For this review, use the dimensioned drawing (mm, ordinates from the lowest corner) and the shaded views. Give positions to 0.01 mm unless a question says otherwise; leave off trailing zeros. Write each loop counter-clockwise with the first axis right and the second up, starting at its lowest first coordinate (ties: lowest second). Pieces come first, ordered by that corner, then holes. Notation, with made-up numbers: M 16,14 L 24,14 A26 cw 24,43 Z; hole C 87.25,13 d9. An arc over 180 degrees is marked long. Use a Markdown table: item, result. Add a question column.
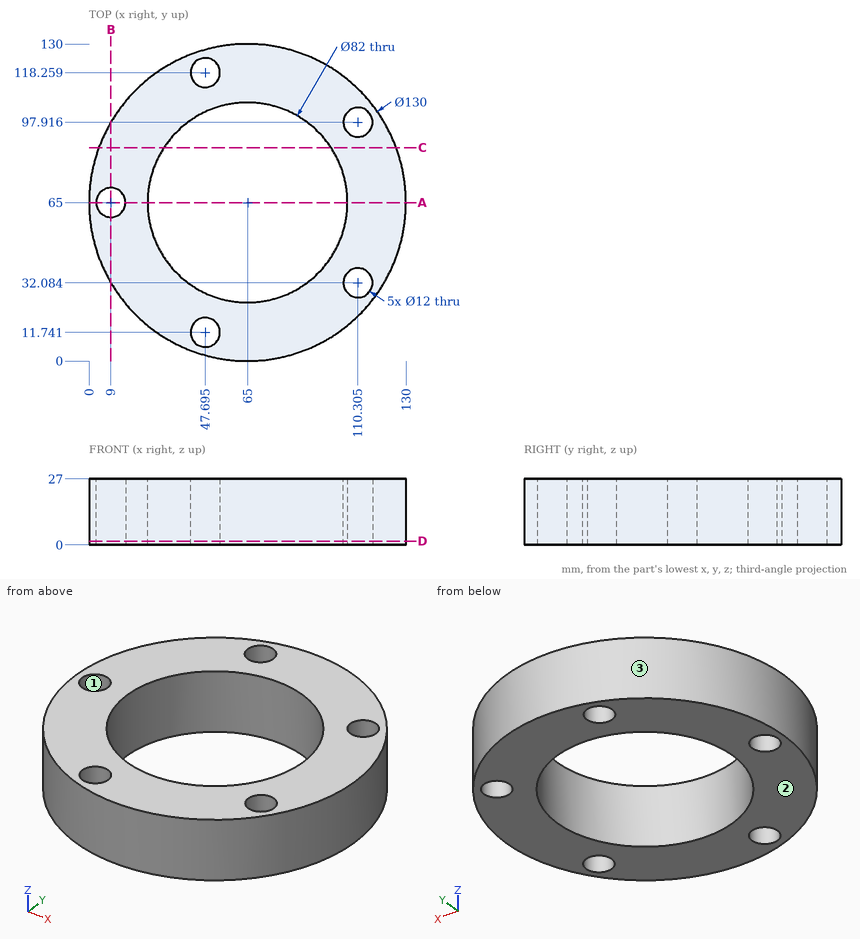
(1) Add section B-B on x = 9. Give the boundary of the cut face in (y, z), then the cut area to 3 significant figures.
(2) Add section C-C on y = 87.5. Give the boundary of the cut face in (x, z), then the cut area to 3 significant figures.
(3) Add section D-D on z = 1.5. Give the boundary of the cut face in (x, y) (1 decimal), then the cut area to 3 significant figures.
(4) Add section A-A on y = 65. Give the boundary of the cut face in (x, z).
(5) The part is to be moulded in two halves that separate along Y. For the marked faces 1, 2 and 3, say which applies: released by +Y, released by -Y, zero draft, split by the parting line, or undercut.
(6) For pin 1 (12 mm diameter, centred on x = 61.5, z = 9.5, fed in from -Y); pin 2 (2 mm diameter, centred on y = 32.5, z = 4, fed in from -X); pin 3 (10 mm diameter, centred on x = 35, z = 4.5, fed in from -Y), all flat-tipped, find the tip position at first contact; note any pin that passes through.
(7) Wall thickness on L1, parallel to Y at x = 64, z = 16.5; L2, parallel to Y at x = 43, z = 25.5 (1 decimal); L3, parallel to X at y = 70, z = 10.75 (1 decimal): over which ranges is each line inside the solid? List them lowest first.
From the geometry:
| question | item | result |
|---|---|---|
| 1 | outline | M 32,0 L 59,0 L 59,27 L 32,27 Z; M 71,0 L 98,0 L 98,27 L 71,27 Z |
| 1 | area | 1,460 mm^2 |
| 2 | outline | M 4.02,0 L 30.73,0 L 30.73,27 L 4.02,27 Z; M 99.27,0 L 125.98,0 L 125.98,27 L 99.27,27 Z |
| 2 | area | 1,440 mm^2 |
| 3 | outline | C 65,65 d130; hole C 9,65 d12; hole C 65,65 d82; hole C 47.7,11.7 d12; hole C 47.7,118.3 d12; hole C 110.3,32.1 d12; hole C 110.3,97.9 d12 |
| 3 | area | 7,430 mm^2 |
| 4 | outline | M 0,0 L 3,0 L 3,27 L 0,27 Z; M 15,0 L 24,0 L 24,27 L 15,27 Z; M 106,0 L 130,0 L 130,27 L 106,27 Z |
| 5 | face 1 | undercut |
| 5 | face 2 | zero draft |
| 5 | face 3 | split by the parting line |
| 6 | pin 1 | stops at y = 0 |
| 6 | pin 2 | stops at x = 8.14 |
| 6 | pin 3 | stops at y = 5 |
| 7 | L1 | y = 0.01 to 24.01, 105.99 to 129.99 |
| 7 | L2 | y = 3.8 to 8, 15.5 to 30.4, 99.6 to 114.5, 122 to 126.2 |
| 7 | L3 | x = 0.2 to 5.7, 12.3 to 24.3, 105.7 to 129.8 |
